from build123d import *

# Parameters (mm, degrees)
F0_R     = 19.5
F1_DEPTH = 3
F2_DEPTH = 1


# Not quite as in the source:
# - a feature names something its author has since deleted; it is built from what else it names


with BuildPart() as f1:
    # F0 (on Top) → F1 (new body)
    with BuildSketch(Plane.XY):
        with Locations((6.52368e-05, -6.45803e-05)):
            Circle(F0_R)
        with BuildLine():
            ThreePointArc((-8.3389530288, -11.8822470528), (-8.632845655, -11.8822470528), (-8.723663471, -11.6027385556))
            Line((-8.723663471, -11.6027385556), (-5.5384419263, -1.7996346453))
            Line((-5.5384419263, -1.7996346453), (-13.877460192, 4.2590167665))
            ThreePointArc((-13.877460192, 4.2590167665), (-13.968278008, 4.5385252636), (-13.7305138789, 4.7112710151))
            Line((-13.7305138789, 4.7112710151), (-3.4229204369, 4.7112710151))
            Line((-3.4229204369, 4.7112710151), (-0.2376988922, 14.5143749254))
            ThreePointArc((-0.2376988922, 14.5143749254), (6.52368e-05, 14.6871206768), (0.2378293659, 14.5143749254))
            Line((0.2378293659, 14.5143749254), (3.4230509106, 4.7112710151))
            Line((3.4230509106, 4.7112710151), (13.7306443525, 4.7112710151))
            ThreePointArc((13.7306443525, 4.7112710151), (13.9684084816, 4.5385252637), (13.8775906656, 4.2590167665))
            Line((13.8775906656, 4.2590167665), (5.5385724, -1.7996346453))
            Line((5.5385724, -1.7996346453), (8.7237939446, -11.6027385556))
            ThreePointArc((8.7237939446, -11.6027385556), (8.6329761286, -11.8822470528), (8.3390835025, -11.8822470528))
            Line((8.3390835025, -11.8822470528), (6.52368e-05, -5.823595641))
            Line((6.52368e-05, -5.823595641), (-8.3389530288, -11.8822470528))
        make_face(mode=Mode.SUBTRACT)
    extrude(amount=F1_DEPTH)

    # F0 (on Top) → F2 (join)
    with BuildSketch(Plane.XY):
        with BuildLine():
            Line((-5.5384419263, -1.7996346453), (-8.723663471, -11.6027385556))
            ThreePointArc((-8.723663471, -11.6027385556), (-8.632845655, -11.8822470528), (-8.3389530288, -11.8822470528))
            Line((-8.3389530288, -11.8822470528), (6.52368e-05, -5.823595641))
            Line((6.52368e-05, -5.823595641), (-5.5384419263, -1.7996346453))
        make_face()
        with BuildLine():
            Line((-13.877460192, 4.2590167665), (-5.5384419263, -1.7996346453))
            Line((-5.5384419263, -1.7996346453), (-3.4229204369, 4.7112710151))
            Line((-3.4229204369, 4.7112710151), (-13.7305138789, 4.7112710151))
            ThreePointArc((-13.7305138789, 4.7112710151), (-13.968278008, 4.5385252636), (-13.877460192, 4.2590167665))
        make_face()
        Polygon((-3.4229204369, 4.7112710151), (-5.5384419263, -1.7996346453), (6.52368e-05, -5.823595641), (5.5385724, -1.7996346453), (3.4230509106, 4.7112710151), align=None)
        with BuildLine():
            Line((-0.2376988922, 14.5143749254), (-3.4229204369, 4.7112710151))
            Line((-3.4229204369, 4.7112710151), (3.4230509106, 4.7112710151))
            Line((3.4230509106, 4.7112710151), (0.2378293659, 14.5143749254))
            ThreePointArc((0.2378293659, 14.5143749254), (6.52368e-05, 14.6871206768), (-0.2376988922, 14.5143749254))
        make_face()
        with BuildLine():
            Line((5.5385724, -1.7996346453), (6.52368e-05, -5.823595641))
            Line((6.52368e-05, -5.823595641), (8.3390835025, -11.8822470528))
            ThreePointArc((8.3390835025, -11.8822470528), (8.6329761286, -11.8822470528), (8.7237939446, -11.6027385556))
            Line((8.7237939446, -11.6027385556), (5.5385724, -1.7996346453))
        make_face()
        with BuildLine():
            Line((13.7306443525, 4.7112710151), (3.4230509106, 4.7112710151))
            Line((3.4230509106, 4.7112710151), (5.5385724, -1.7996346453))
            Line((5.5385724, -1.7996346453), (13.8775906656, 4.2590167665))
            ThreePointArc((13.8775906656, 4.2590167665), (13.9684084816, 4.5385252637), (13.7306443525, 4.7112710151))
        make_face()
    extrude(amount=F2_DEPTH)


solid = f1.part
Input: part model. Units: mm. Frame: model coordinates. A direction names the side the tool comes from. Give positions to 0.01 mm unless a question says otherwise; leave off trailing zeros. Loops run counter-clockwise (first coordinate to the right, second up) from the corner with the lowest first, then second, coordinate; pieces in that order, holes last. Notation, with made-up numbers: M 11,62 L 60,62 A15 ccw 60,74 Z; hole C 24.5,-11 d3. An arc over 180 degrees is marked long. Use one line per item in the form item = value.
1. Section query D-D, the plane x = -6.5. Return the cut outline in (y, z).
Numbers:
outline = M -18.38,0 L 18.38,0 L 18.38,3 L 4.71,3 L 4.71,1 L -1.1,1 L -1.1,3 L -4.76,3 L -4.76,1 L -10.55,1 L -10.55,3 L -18.38,3 Z
2. Section query C-C, the plane z = 1.8. Return the cut outline in (x, y), and give its area (3 significant figures).
Numbers:
outline = C 0,0 d39; hole M -13.88,4.26 L -5.54,-1.8 L -8.72,-11.6 A0.25 ccw -8.34,-11.88 L 0,-5.82 L 8.34,-11.88 A0.25 ccw 8.72,-11.6 L 5.54,-1.8 L 13.88,4.26 A0.25 ccw 13.73,4.71 L 3.42,4.71 L 0.24,14.51 A0.25 ccw -0.24,14.51 L -3.42,4.71 L -13.73,4.71 A0.25 ccw Z
area = 934 mm²
3. Section query A-A, the plane y = -8.5. Return the cut outline in (x, z), and give its area (3 significant figures).
Numbers:
outline = M -17.55,0 L 17.55,0 L 17.55,3 L 7.72,3 L 7.72,1 L 3.68,1 L 3.68,3 L -3.68,3 L -3.68,1 L -7.72,1 L -7.72,3 L -17.55,3 Z
area = 89.2 mm²
4. First-contact query: pin 1 (1.5 mm diameter, centred on y = 9.5, z = 1, fed in from -X); pin 2 (1 mm diameter, centred on x = 11, z = 2, fed in from -Y); pin 3 (1.5 mm diameter, centred on y = -13.5, z = 2.5, fed in from -X). Flat tips, straight axial feed; report the tip coordinate or a pass-through.
Numbers:
pin_1 = -17.43
pin_2 = -16.43
pin_3 = -14.75
5. Line query: L1, parallel to X at y = -10, z = 1.55; L2, parallel to X at y = -11, z = 1.55; L3, parallel to Y at x = -5, z = 2.05. Output: solid intervals per line, ascending.
Numbers:
L1 = -16.74 to -8.2, -5.75 to 5.75, 8.2 to 16.74
L2 = -16.1 to -8.53, -7.12 to 7.12, 8.53 to 16.1
L3 = -18.85 to -9.46, 4.71 to 18.85
6. Pull-direction query (X, two-part tool) for faces 3 (the face through (7.1, -6.6, 2)), 4 (the face through (-4.227, -19.036, 1.479)), 5 (the face through (0, 0, 0)); classes: released by +X, released by -X, zero draft, split by the parting line, or undercut.
Numbers:
face_3 = undercut
face_4 = split by the parting line
face_5 = zero draft
7. Reachability of faces 1 (the face through (0, -8, 3)), 2 (the face through (-1.853, 9.544, 1.986)) from +Z, -Z, +X, -X, +Y, -Y: full face, straight path, thin tool, end or side. Return the list, or none.
Numbers:
face_1 = +Z, +X, -X, +Y, -Y
face_2 = +Z
8. Section query B-B, the plane x = 10.5. Return the cut outline in (y, z).
Numbers:
outline = M -16.43,0 L 16.43,0 L 16.43,3 L 4.71,3 L 4.71,1 L 1.81,1 L 1.81,3 L -16.43,3 Z
